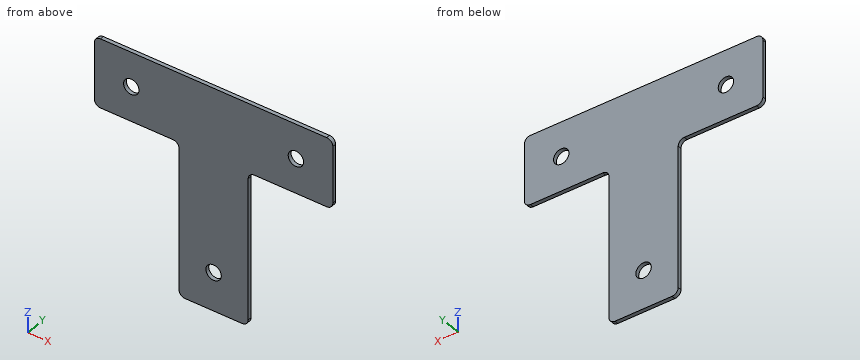
from build123d import *

# Parameters (mm, degrees)
F0_R     = 5
F1_DEPTH = 2.5


with BuildPart() as f1:
    # F0 (on Front) → F1 (new body)
    with BuildSketch(Plane.XZ):
        with BuildLine():
            ThreePointArc((77.5, 18.5), (76.328427, 21.328427), (73.5, 22.5))
            Line((73.5, 22.5), (-73.5, 22.5))
            ThreePointArc((-73.5, 22.5), (-76.328427, 21.328427), (-77.5, 18.5))
            Line((-77.5, 18.5), (-77.5, -18.5))
            ThreePointArc((-77.5, -18.5), (-76.328427, -21.328427), (-73.5, -22.5))
            Line((-73.5, -22.5), (-26.5, -22.5))
            Line((-26.5, -22.5), (22.5, -22.5))
            Line((22.5, -22.5), (26.5, -22.5))
            Line((26.5, -22.5), (73.5, -22.5))
            ThreePointArc((73.5, -22.5), (76.328427, -21.328427), (77.5, -18.5))
            Line((77.5, -18.5), (77.5, 18.5))
        make_face()
        with Locations((-53.5, 0)):
            Circle(F0_R, mode=Mode.SUBTRACT)
        with Locations((53.5, 0)):
            Circle(F0_R, mode=Mode.SUBTRACT)
        with BuildLine():
            ThreePointArc((22.5, -26.5), (23.671573, -23.671573), (26.5, -22.5))
            Line((26.5, -22.5), (22.5, -22.5))
            Line((22.5, -22.5), (-26.5, -22.5))
            ThreePointArc((-26.5, -22.5), (-23.671573, -23.671573), (-22.5, -26.5))
            Line((-22.5, -26.5), (-22.5, -118.5))
            ThreePointArc((-22.5, -118.5), (-21.328427, -121.328427), (-18.5, -122.5))
            Line((-18.5, -122.5), (18.5, -122.5))
            ThreePointArc((18.5, -122.5), (21.328427, -121.328427), (22.5, -118.5))
            Line((22.5, -118.5), (22.5, -26.5))
        make_face()
        with Locations((0, -97.5)):
            Circle(F0_R, mode=Mode.SUBTRACT)
    extrude(amount=F1_DEPTH)


solid = f1.part
Work out the finished part from the listing and answer in its coordinate system (mm). Coordinates: 2 decimals unless noted, no trailing zeros. Loops run counter-clockwise (first coordinate to the right, second up) from the corner with the lowest first, then second, coordinate; pieces in that order, holes last. Notation, with made-up numbers: M 53.25,-24.75 L 79.25,-24.75 A21 cw 79.25,4.25 Z; hole C 25,-34 d8. An arc over 180 degrees is marked long. Answer in a Markdown table with one row per item. Add a question column.
1. Consider L1, parallel to Z at x = -53, y = -1.75; L2, parallel to Z at x = 0, y = -0.9; L3, parallel to X at y = -0.7, z = -44. Determine where each line is inside the solid, lowest interval first.
2. Find section D-D, the plane x = 0. Write down the section's boundary in (y, z).
3. Find section B-B, the plane z = 0. Write down the section's boundary in (x, y), then the cut area to 4 significant figures.
4. Find section C-C, the plane y = -2.05. Write down the section's boundary in (x, z), then the cut area to 3 significant figures.
5. Find section A-A, the plane x = 53.5. Write down the section's boundary in (y, z).
6. Flat-ended cylindrical pins translate along their axes: P1, Ø1.2, axis at y = -1.5, z = -52, coming from the +X side; P2, Ø1.2, axis at x = -40, y = -1, coming from the -Z side. Find the tip coordinate at first contact, or state that the pin passes through.
Reported:
| question | item | result |
|---|---|---|
| 1 | L1 | z = -22.5 to -4.97, 4.97 to 22.5 |
| 1 | L2 | z = -122.5 to -102.5, -92.5 to 22.5 |
| 1 | L3 | x = -22.5 to 22.5 |
| 2 | outline | M -2.5,-122.5 L 0,-122.5 L 0,-102.5 L -2.5,-102.5 Z; M -2.5,-92.5 L 0,-92.5 L 0,22.5 L -2.5,22.5 Z |
| 3 | outline | M -77.5,-2.5 L -58.5,-2.5 L -58.5,0 L -77.5,0 Z; M -48.5,-2.5 L 48.5,-2.5 L 48.5,0 L -48.5,0 Z; M 58.5,-2.5 L 77.5,-2.5 L 77.5,0 L 58.5,0 Z |
| 3 | area | 337.5 mm^2 |
| 4 | outline | M -77.5,-18.5 A4 ccw -73.5,-22.5 L -26.5,-22.5 A4 cw -22.5,-26.5 L -22.5,-118.5 A4 ccw -18.5,-122.5 L 18.5,-122.5 A4 ccw 22.5,-118.5 L 22.5,-26.5 A4 cw 26.5,-22.5 L 73.5,-22.5 A4 ccw 77.5,-18.5 L 77.5,18.5 A4 ccw 73.5,22.5 L -73.5,22.5 A4 ccw -77.5,18.5 Z; hole C -53.5,0 d10; hole C 0,-97.5 d10; hole C 53.5,0 d10 |
| 4 | area | 11,200 mm^2 |
| 5 | outline | M -2.5,-22.5 L 0,-22.5 L 0,-5 L -2.5,-5 Z; M -2.5,5 L 0,5 L 0,22.5 L -2.5,22.5 Z |
| 6 | P1 | stops at x = 22.5 |
| 6 | P2 | stops at z = -22.5 |
